Geometry check sheet. Reference: the model listing, model coordinates, mm. Give positions to 0.01 mm unless a question says otherwise; leave off trailing zeros. Order: outer loops, then holes, each group sorted by start corner. A loop starts at its lowest first (then second) coordinate and runs counter-clockwise, first axis right, second up. Notation, with made-up numbers: M 23.5,-36 L 38.5,-36 A14 cw 38.5,-26 Z; hole C 74,9.25 d8. An arc over 180 degrees is marked long. Answer as CSV lines item,"result". Start each with the question number.
Q1. Section check A-A, the plane x = 0. Record the boundary of the cut face in (y, z), then the cut area to 3 significant figures.
Q2. Section check D-D, the plane z = 4. Record the boundary of the cut face in (x, y).
Q3. Thickness scan on line 1 (X direction, y = 0.4, z = 1); line 2 (Z direction, x = 4, y = 2); line 3 (Z direction, x = -4.5, y = 1). Record the ranges inside material, lowest first.
Q4. Section check B-B, the plane z = 0. Record the boundary of the cut face in (x, y), then the cut area to 3 significant figures.
Q5. Go/stop test with flat-tipped pins: pin 1 (1.5 mm diameter, centred on x = 9, y = 3.5, fed in from -Z); pin 2 (1 mm diameter, centred on y = 1.5, z = 5.5, fed in from -X); pin 3 (3 mm diameter, centred on y = 4, z = 9.5, fed in from +X). Record where each tip stops, or that it passes through.
Q6. Mould release check, pull along X, two halves, no side actions. Record for faces 1 (the cylindrical face through (10.5, 2.46, -0.07)), 2 (the flat face through (0, 5, 6)), 3 (the cylindrical face through (-12.544, 2.465, -2.786)): +X half, -X half, draft (parallel to the pull), parting line (faces both ways), or undercut.
Q7. Section check C-C, the plane x = -4.5. Record the boundary of the cut face in (y, z), then the cut area to 3 significant figures.
```python
from build123d import *

# Parameters (mm, degrees)
SKETCH1_R             = 12.85
SKETCH1_R_2           = 1.5
SKETCH1_R_3           = 5
BOSS_EXTRUDE1_DEPTH   = 5
F_6_0MM_DOWEL_HOLE1_D = 3


with BuildPart() as part:
    # Sketch1 → Boss-Extrude1 (new body)
    with BuildSketch(Plane(origin=(0, 0, 0), x_dir=(1, 0, 0), z_dir=(0, 1, 0))):
        with Locations(Location((0, 0, 0), (0, 0, 270))):
            Circle(SKETCH1_R)
        with Locations(Location((4.5, 7.794228634, 0), (0, 0, 270))):
            Circle(SKETCH1_R_2, mode=Mode.SUBTRACT)
        with Locations(Location((-9, 0, 0), (0, 0, 270))):
            Circle(SKETCH1_R_2, mode=Mode.SUBTRACT)
        with Locations(Location((4.5, -7.794228634, 0), (0, 0, 270))):
            Circle(SKETCH1_R_2, mode=Mode.SUBTRACT)
        with Locations(Location((0, 0, 0), (0, 0, 270))):
            Circle(SKETCH1_R_3, mode=Mode.SUBTRACT)
    extrude(amount=BOSS_EXTRUDE1_DEPTH)

    # Ø6.0mm Dowel Hole1 (through all)
    with Locations(Plane(origin=(0, 5, 0), x_dir=(1, 0, 0), z_dir=(0, 1, 0))):
        with Locations((9, 0), (-4.5, 7.794228634), (-4.5, -7.794228634)):
            Hole(F_6_0MM_DOWEL_HOLE1_D / 2)


solid = part.part
```
Answer block:
1,outline,"M 0,-12.85 L 5,-12.85 L 5,-5 L 0,-5 Z; M 0,5 L 5,5 L 5,12.85 L 0,12.85 Z"
1,area,"78.5 mm2"
2,outline,"M -12.21,0 L -3,0 L -3,5 L -12.21,5 Z; M 3,0 L 12.21,0 L 12.21,5 L 3,5 Z"
3,line 1,"x = -12.81 to -10.12, -7.88 to -4.9, 4.9 to 7.88, 10.12 to 12.81"
3,line 2,"z = -12.21 to -9.21, -6.38 to -3, 3 to 6.38, 9.21 to 12.21"
3,line 3,"z = -12.04 to -9.29, -6.29 to -2.18, 2.18 to 6.29, 9.29 to 12.04"
4,outline,"M -12.85,0 L -10.5,0 L -10.5,5 L -12.85,5 Z; M -7.5,0 L -5,0 L -5,5 L -7.5,5 Z; M 5,0 L 7.5,0 L 7.5,5 L 5,5 Z; M 10.5,0 L 12.85,0 L 12.85,5 L 10.5,5 Z"
4,area,"48.5 mm2"
5,pin 1,"stops at z = -9.85"
5,pin 2,"stops at x = -11.84"
5,pin 3,"stops at x = 10.06"
6,face 1,"undercut"
6,face 2,"draft"
6,face 3,"parting line"
7,outline,"M 0,-12.04 L 5,-12.04 L 5,-9.29 L 0,-9.29 Z; M 0,-6.29 L 5,-6.29 L 5,-2.18 L 0,-2.18 Z; M 0,2.18 L 5,2.18 L 5,6.29 L 0,6.29 Z; M 0,9.29 L 5,9.29 L 5,12.04 L 0,12.04 Z"
7,area,"68.6 mm2"
